from build123d import *

# Parameters (mm, degrees)
SKETCH6_R           = 1
BOSS_EXTRUDE1_DEPTH = 3.9


with BuildPart() as part:
    # Sketch6 → Boss-Extrude1 (new body)
    with BuildSketch(Plane.XY):
        with BuildLine():
            Line((24.518959729, 113.266913748), (12.546015233, 94.029173129))
            add(Edge.make_bspline(
                [(12.546015233, 94.029173129), (11.143200975, 90.620780812), (11.195857544, 87.895488842)],
                knots=[0, 0, 0, 1, 1, 1], degree=2))
            ThreePointArc((11.195857544, 87.895488842), (15.023721592, 85.0119769), (16.738951622, 89.486926087))
            add(Edge.make_bspline(
                [(18.016460853, 94.194825281), (15.988617018, 91.415760023), (16.738951622, 89.486926087)],
                knots=[0, 0, 0, 1, 1, 1], degree=2))
            Line((18.016460853, 94.194825281), (29.628743828, 114.037411274))
            ThreePointArc((29.628743828, 114.037411274), (29.791338928, 114.286113373), (29.977739072, 114.517511055))
            ThreePointArc((29.977739072, 114.517511055), (28.402741778, 119.438186194), (24.854741229, 115.682476887))
            ThreePointArc((24.854741229, 115.682476887), (24.943384664, 114.439035131), (24.518959729, 113.266913748))
        make_face()
        with Locations((27.737526551, 116.51286763)):
            Circle(SKETCH6_R, mode=Mode.SUBTRACT)
        with Locations((14.195857544, 87.895488842)):
            Circle(SKETCH6_R, mode=Mode.SUBTRACT)
    extrude(amount=BOSS_EXTRUDE1_DEPTH)


solid = part.part
Verification items for the finished model (mm, model axes). Coordinates: 2 decimals unless noted, no trailing zeros. Order: outer loops, then holes, each group sorted by start corner. A loop starts at its lowest first (then second) coordinate and runs counter-clockwise, first axis right, second up.
Item 1: Material ranges on L1, parallel to X at y = 88, z = 1.3; L2, parallel to X at y = 96, z = 3.55; L3, parallel to Y at x = 27.75, z = 2.7, recorded low to high.
Filled in:
L1: x = 11.19 to 13.2, 15.19 to 17.19
L2: x = 13.77 to 19.07
L3: y = 110.83 to 115.51, 117.51 to 119.51
Item 2: Depth check by flat-ended pin: pin 1 (1 mm diameter, centred on y = 94.5, z = 2.5, fed in from -X). Enter the tip coordinate at first touch or a pass-through.
Filled in:
pin 1: stops at x = 12.53
Item 3: Release check for a two-part mould opening along Y. For faces 1 (the face through (18.616, 103.783, 1.923)), 2 (the face through (27.607, 117.504, 1.923)), 3 (the face through (23.741, 103.977, 1.923)), 4 (the face through (20, 102, 0)) record: +Y half, -Y half, draft (parallel to the pull), parting line (faces both ways), or undercut.
Filled in:
face 1: +Y half
face 2: undercut
face 3: -Y half
face 4: draft
Item 4: Section check D-D, the plane z = 0.4. Give the number of separate pieces and of enclosed holes in the cut face, then the cut area to 3 significant figures.
Filled in:
separate pieces: 1
enclosed holes: 2
area: 168 mm2
Item 5: Section check A-A, the plane x = 14.5. Enter the section's corners in (y, z), then the cut area to 3 significant figures.
Filled in:
outline: (84.91, 0) - (86.94, 0) - (86.94, 3.9) - (84.91, 3.9) - close; (88.85, 0) - (97.17, 0) - (97.17, 3.9) - (88.85, 3.9) - close
area: 40.4 mm2
Item 6: Section check B-B, the plane y = 101.5. Enter the section's corners in (x, z).
Filled in:
outline: (17.2, 0) - (22.29, 0) - (22.29, 3.9) - (17.2, 3.9) - close
Item 7: Section check C-C, the plane x = 28. Enter the section's corners in (y, z), then the cut area to 3 significant figures.
Filled in:
outline: (111.25, 0) - (115.55, 0) - (115.55, 3.9) - (111.25, 3.9) - close; (117.48, 0) - (119.5, 0) - (119.5, 3.9) - (117.48, 3.9) - close
area: 24.6 mm2
